from build123d import *

# Parameters (mm, degrees)
BOSS_EXTRUDE6_DEPTH = 14
SKETCH8_R           = 3.68
CUT_EXTRUDE1_DEPTH  = 10
SKETCH10_W          = 31.702507637
SKETCH10_H          = 2.761891862
BOSS_EXTRUDE8_DEPTH = 50
FILLET2_R           = 5


with BuildPart() as part:
    # Sketch7 → Boss-Extrude6 (new body)
    with BuildSketch(Plane(origin=(0, 0, 44.491647423), x_dir=(0, 1, 0), z_dir=(1, 0, 0))):
        Polygon((57.244330768, -80.05237461), (75.978257712, -80.05237461), (75.978257712, -82.841498661), (83.21636585, -82.841498661), (83.21636585, -107.310582048), (85.978257712, -107.310582048), (85.978257712, -75.608074412), (57.244330768, -75.608074412), align=None)
    extrude(amount=-BOSS_EXTRUDE6_DEPTH)

    # Sketch8 → Cut-Extrude1 (cut)
    with BuildSketch(Plane.XY.offset(-31.116426988)):
        with Locations((-6.819274641, 63.278257712)):
            Circle(SKETCH8_R)
    extrude(amount=-CUT_EXTRUDE1_DEPTH, mode=Mode.SUBTRACT)

    # Sketch10 → Boss-Extrude8 (add)
    with BuildSketch(Plane.ZY.offset(14)):
        with Locations((-46.967680806, 84.597311781)):
            Rectangle(SKETCH10_W, SKETCH10_H)
    extrude(amount=BOSS_EXTRUDE8_DEPTH)

    # Fillet2
    fillet2_edges = [part.edges().sort_by_distance(p)[0] for p in [
        (-64, 84.597311781, -62.818934625),
        (0, 84.597311781, -62.818934625),
        (0, 57.244330768, -33.338577087),
        (-14, 57.244330768, -33.338577087),
        (-64, 84.597311781, -31.116426988),
        (-14, 83.21636585, -34.733139113),
    ]]
    fillet(fillet2_edges, radius=FILLET2_R)


solid = part.part
Geometry check sheet. Reference: the model listing, model coordinates, mm. A direction names the side the tool comes from. Coordinates: 2 decimals unless noted, no trailing zeros. Order: outer loops, then holes, each group sorted by start corner. A loop starts at its lowest first (then second) coordinate and runs counter-clockwise, first axis right, second up. Notation, with made-up numbers: M 71.5,-27.5 L 111.5,-27.5 A10 ccw 111.5,-20.5 Z; hole C 85.25,-14 d9. An arc over 180 degrees is marked long. Use CSV: the item, a comma, the result in double quotes.
Item 1: Cross-section at B-B on x = -12.5. Record the cut outline in (y, z).
Returned:
outline,"M 58.67,-35.56 L 75.98,-35.56 L 75.98,-38.35 L 83.22,-38.35 L 83.22,-62.82 L 85.98,-62.82 L 85.98,-31.12 L 58.67,-31.12 Z"
Item 2: Cross-section at C-C on z = -45. Record the cut outline in (x, y), then the cut area to 3 significant figures.
Returned:
outline,"M -64,83.22 L 0,83.22 L 0,85.98 L -64,85.98 Z"
area,"177 mm2"
Item 3: Tool access check on faces 1 (the flat face through (-32, 83.216, -47)), 2 (the flat face through (-32, 85, -62.819)), 3 (the flat face through (-7, 80, -38.35)), 4 (the flat face through (-12, 77, -31.116)), 5 (the flat face through (-14, 70, -34)). Record the directions out of +Z, -Z, +X, -X, +Y, -Y that give a thin tool (end or side, any length) a straight path to the whole face; none if there is none.
Returned:
face 1,"-Z, -X, -Y"
face 2,"-Z, +X, -X, +Y, -Y"
face 3,"-Z, +X, -X, -Y"
face 4,"+Z, +X, -X, +Y, -Y"
face 5,"+Z, -Z, -X, -Y"
Item 4: Cross-section at A-A on y = 61.25. Record the cut outline in (x, z), then the cut area to 3 significant figures.
Returned:
outline,"M -13.9,-35.56 L -9.89,-35.56 L -9.89,-31.12 L -13.9,-31.12 Z; M -3.75,-35.56 L -0.1,-35.56 L -0.1,-31.12 L -3.75,-31.12 Z"
area,"34.0 mm2"
Item 5: Thickness scan on line 1 along Y through (x, z) = (-47.5, -40.5); line 2 along Z through (x, y) = (-11, 61); line 3 along X through (y, z) = (59.25, -34). Record the ranges inside material, lowest first.
Returned:
line 1,"y = 83.22 to 85.98"
line 2,"z = -35.56 to -31.12"
line 3,"x = -13 to -1"
Item 6: Cross-section at D-D on y = 76.75. Record the cut outline in (x, z).
Returned:
outline,"M -14,-38.35 L 0,-38.35 L 0,-31.12 L -14,-31.12 Z"
Item 7: Gauge pin test, flat ends, axial feed: pin 1 Ø15.5 at (x, y) = (-5, 71) entering from -Z; pin 2 Ø3.5 at (y, z) = (66.5, -35.5) entering from -X; pin 3 Ø12 at (x, y) = (-6.82, 63.28) entering from -Z. Record the tip position at first contact, or that the pin passes through.
Returned:
pin 1,"stops at z = -38.35"
pin 2,"stops at x = -14"
pin 3,"stops at z = -35.56"
Item 8: Mould release check, pull along X, two halves, no side actions. Record for faces 6 (the cylindrical face through (-7.298, 66.927, -33.307)), 7 (the flat face through (-7, 69, -35.561)), 8 (the cylindrical face through (-62.574, 84.617, -32.62)): pulls with the +X half, pulls with the -X half, needs draft (parallel to the pull), parting line crosses it, or undercut.
Returned:
face 6,"undercut"
face 7,"needs draft"
face 8,"pulls with the -X half"
